Could you check a few things on this drawing? It's one solid part, dimensions in mm from its lowest x, y, z. A direction names the side the tool comes from. Round coordinates to 2 decimals unless told otherwise and drop trailing zeros. Loops run counter-clockwise (first coordinate to the right, second up) from the corner with the lowest first, then second, coordinate; pieces in that order, holes last. Notation, with made-up numbers: (-28.75, 16) -> (-24.75, 16) arc R19 ccw to (-24.75, 26) -> close; hole circle Ø7 at (-29.5, -17.5). An arc over 180 degrees is marked (long way). Put each result on its own line as item: value. Start each with the question number.
1. Imagine slicing it at A-A, the plane y = 16.25. Please give me the cut outline in (x, z) (1 decimal), and give its area (3 significant figures).
2. Imagine slicing it at D-D, the plane z = 7.75. Please give me the cut outline in (x, y).
3. Which directions (+Z, -Z, +X, -X, +Y, -Y) give clear straight access to the entire face, cutting with the end or side of a thin tool? Please do the marked faces 4 and 5.
4. Imagine slicing it at B-B, the plane x = 7. Please give me the cut outline in (y, z) (1 decimal).
5. I need wall thicknesses on line 1 (Y direction, x = 1.75, z = 4); line 2 (X direction, y = 13, z = 6.25) (1 decimal); line 3 (X direction, y = 5, z = 5) (1 decimal). Which ranges of each line are inside material? Lowest first, please. Write a range as [from, to].
6. I'm going to push flat-ended pins straight in: P1, Ø5, axis at y = 3, z = 7, coming from the +X side; P2, Ø1, axis at y = 2.5, z = 2.5, coming from the -X side. Where does each tip first touch, or does it pass through?
7. If we mould it in two halves opening along Y, with no side actions, what happens to the marked faces 1, 2 and 3? For each: pulls with the +Y half, pulls with the -Y half, needs draft (parallel to the pull), parting line crosses it, or undercut.
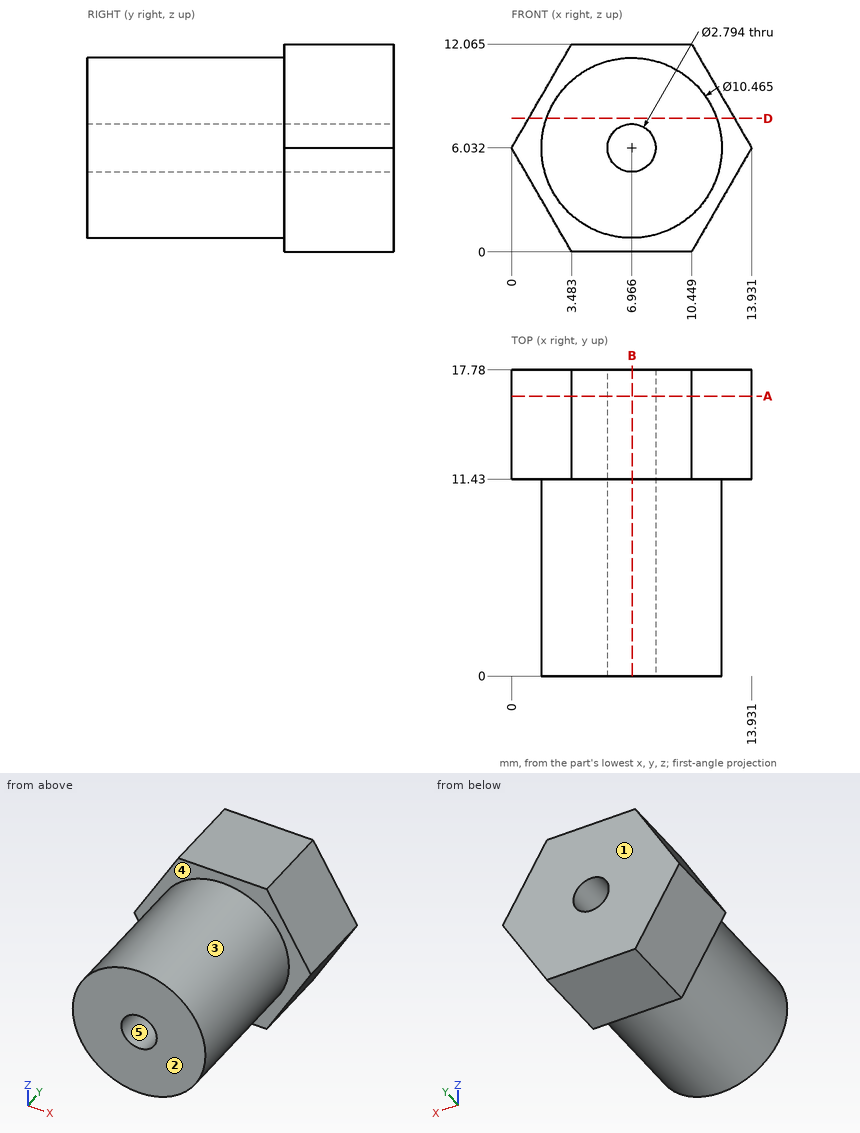
Entries:
1. outline: (0, 6) -> (3.5, 0) -> (10.4, 0) -> (13.9, 6) -> (10.4, 12.1) -> (3.5, 12.1) -> close; hole circle Ø2.8 at (7, 6)
1. area: 120 mm^2
2. outline: (0.99, 11.43) -> (2.02, 11.43) -> (2.02, 0) -> (11.91, 0) -> (11.91, 11.43) -> (12.94, 11.43) -> (12.94, 17.78) -> (0.99, 17.78) -> close
3. face 4: -Y
3. face 5: +Y, -Y
4. outline: (0, 0.8) -> (11.4, 0.8) -> (11.4, 0) -> (17.8, 0) -> (17.8, 4.6) -> (0, 4.6) -> close; (0, 7.4) -> (17.8, 7.4) -> (17.8, 12.1) -> (11.4, 12.1) -> (11.4, 11.3) -> (0, 11.3) -> close
5. line 1: [11.43, 17.78]
5. line 2: [0.1, 5.6], [8.3, 13.8]
5. line 3: [1.8, 6], [7.9, 12.1]
6. P1: x = 12.2
6. P2: x = 2.7
7. face 1: pulls with the +Y half
7. face 2: pulls with the -Y half
7. face 3: needs draft
